Here's how the part is built. I have some questions about the finished solid (model axes, mm). A direction names the side the tool comes from. Coordinates: 2 decimals unless noted, no trailing zeros. Loops run counter-clockwise (first coordinate to the right, second up) from the corner with the lowest first, then second, coordinate; pieces in that order, holes last. Notation, with made-up numbers: (1.25, 12.5) -> (13.25, 12.5) arc R32 ccw to (13.25, 38.5) -> close; hole circle Ø1 at (-39.75, -39.5). An arc over 180 degrees is marked (long way). Answer as a JSON object with one key per item and string values. Group by question number.
1) Which directions (+Z, -Z, +X, -X, +Y, -Y) give clear straight access to the entire face, cutting with the end or side of a thin tool? Please do faces 1 (the flat face through (2.25, -4.39, 4.93)), 2 (the flat face through (2.4, -1.2, 0)).
2) I want a section at A-A (x = 4.5). Write out the boundary of the cut face in (y, z).
3) I want a section at B-B (y = -5.75). Write out the boundary of the cut face in (x, z).
4) I need wall thicknesses on probe 1 along Y at (x, z) = (-1.75, 1.25); probe 2 along Y at (x, z) = (-1.5, 1.5); probe 3 along X at (y, z) = (6.5, 3.5). Which ranges of each line are inside material? Lowest first, please. Write a range as [from, to].
5) If we mould it in two halves opening along Y, with no side actions, what happens to faces 3 (the flat face through (-4.625, -1.483, 4.93)), 4 (the flat face through (2.4, -1.2, 10))? For each: +Y half, -Y half, draft (parallel to the pull), parting line (faces both ways), or undercut.
6) I'm going to push flat-ended pins straight in: pin 1 (5 mm diameter, centred on y = 6, z = 7.5, fed in from +X); pin 2 (5 mm diameter, centred on x = 1.5, y = -2.5, fed in from +Z); pin 3 (4 mm diameter, centred on x = 3, z = 7.5, fed in from +Y); pin 4 (4 mm diameter, centred on x = 2.5, z = 5.5, fed in from -Y). Where does each tip first touch, or does it pass through?
```python
from build123d import *

# Parameters (mm, degrees)
F1_DEPTH = 10


with BuildPart() as f1:
    # F0 (on Top) → F1 (new body)
    with BuildSketch(Plane.XY):
        with BuildLine():
            ThreePointArc((8.3, 0), (5.868986, 5.868986), (0, 8.3))
            ThreePointArc((0, 8.3), (-5.868986, 5.868986), (-8.3, 0))
            ThreePointArc((-8.3, 0), (-5.868986, -5.868986), (0, -8.3))
            ThreePointArc((0, -8.3), (5.868986, -5.868986), (8.3, 0))
        make_face()
        with BuildLine():
            ThreePointArc((-2.496489, 7.072308), (-1.26643, 7.392304), (0, 7.5))
            ThreePointArc((0, 7.5), (1.26643, 7.392304), (2.496489, 7.072308))
            Line((2.496489, 7.072308), (0.497207, 2.245615))
            ThreePointArc((0.497207, 2.245615), (0.880172, 2.124923), (1.236311, 1.939468))
            Line((1.236311, 1.939468), (3.235593, 6.766161))
            ThreePointArc((3.235593, 6.766161), (5.303301, 5.303301), (6.766161, 3.235593))
            Line((6.766161, 3.235593), (1.939468, 1.236311))
            ThreePointArc((1.939468, 1.236311), (2.124923, 0.880172), (2.245615, 0.497207))
            Line((2.245615, 0.497207), (7.072308, 2.496489))
            ThreePointArc((7.072308, 2.496489), (7.392304, 1.26643), (7.5, 0))
            ThreePointArc((7.5, 0), (7.392304, -1.26643), (7.072308, -2.496489))
            Line((7.072308, -2.496489), (2.245615, -0.497207))
            ThreePointArc((2.245615, -0.497207), (2.124923, -0.880172), (1.939468, -1.236311))
            Line((1.939468, -1.236311), (6.766161, -3.235593))
            ThreePointArc((6.766161, -3.235593), (5.303301, -5.303301), (3.235593, -6.766161))
            Line((3.235593, -6.766161), (1.236311, -1.939468))
            ThreePointArc((1.236311, -1.939468), (0.880172, -2.124923), (0.497207, -2.245615))
            Line((0.497207, -2.245615), (2.496489, -7.072308))
            ThreePointArc((2.496489, -7.072308), (1.26643, -7.392304), (0, -7.5))
            ThreePointArc((0, -7.5), (-1.26643, -7.392304), (-2.496489, -7.072308))
            Line((-2.496489, -7.072308), (-0.497207, -2.245615))
            ThreePointArc((-0.497207, -2.245615), (-0.880172, -2.124923), (-1.236311, -1.939468))
            Line((-1.236311, -1.939468), (-3.235593, -6.766161))
            ThreePointArc((-3.235593, -6.766161), (-5.303301, -5.303301), (-6.766161, -3.235593))
            Line((-6.766161, -3.235593), (-1.939468, -1.236311))
            ThreePointArc((-1.939468, -1.236311), (-2.124923, -0.880172), (-2.245615, -0.497207))
            Line((-2.245615, -0.497207), (-7.072308, -2.496489))
            ThreePointArc((-7.072308, -2.496489), (-7.392304, -1.26643), (-7.5, 0))
            ThreePointArc((-7.5, 0), (-7.392304, 1.26643), (-7.072308, 2.496489))
            Line((-7.072308, 2.496489), (-2.245615, 0.497207))
            ThreePointArc((-2.245615, 0.497207), (-2.124923, 0.880172), (-1.939468, 1.236311))
            Line((-1.939468, 1.236311), (-6.766161, 3.235593))
            ThreePointArc((-6.766161, 3.235593), (-5.303301, 5.303301), (-3.235593, 6.766161))
            Line((-3.235593, 6.766161), (-1.236311, 1.939468))
            ThreePointArc((-1.236311, 1.939468), (-0.880172, 2.124923), (-0.497207, 2.245615))
            Line((-0.497207, 2.245615), (-2.496489, 7.072308))
        make_face(mode=Mode.SUBTRACT)
    extrude(amount=F1_DEPTH)


solid = f1.part
```
Determined:
{
 "1": {"face 1": "+Z, -Z", "face 2": "-Z, +X, -X, +Y, -Y"},
 "2": {"outline": "(-6.97, 0) -> (-6, 0) -> (-6, 10) -> (-6.97, 10) -> close; (-2.3, 0) -> (-1.43, 0) -> (-1.43, 10) -> (-2.3, 10) -> close; (1.43, 0) -> (2.3, 0) -> (2.3, 10) -> (1.43, 10) -> close; (6, 0) -> (6.97, 0) -> (6.97, 10) -> (6, 10) -> close"},
 "3": {"outline": "(-5.99, 0) -> (-4.82, 0) -> (-4.82, 10) -> (-5.99, 10) -> close; (-2.81, 0) -> (-1.95, 0) -> (-1.95, 10) -> (-2.81, 10) -> close; (1.95, 0) -> (2.81, 0) -> (2.81, 10) -> (1.95, 10) -> close; (4.82, 0) -> (5.99, 0) -> (5.99, 10) -> (4.82, 10) -> close"},
 "4": {"probe 1": "[-8.11, -7.29], [-5.27, -3.18], [3.18, 5.27], [7.29, 8.11]", "probe 2": "[-8.16, -7.35], [-4.67, -2.58], [2.58, 4.67], [7.35, 8.16]", "probe 3": "[-5.16, -3.74], [-3.13, -2.26], [2.26, 3.13], [3.74, 5.16]"},
 "5": {"face 3": "undercut", "face 4": "draft"},
 "6": {"pin 1": "x = 7.53", "pin 2": "z = 10", "pin 3": "y = 8.24", "pin 4": "y = -8.28"}
}
